```python
from build123d import *

# Parameters (mm, degrees)
F0_W         = 30
F0_H         = 10
F1_DEPTH     = 10
F2_R         = 1.75
F3_DEPTH     = 8
F4_R         = 1.75
F5_DEPTH     = 8
F6_R         = 0.5
F7_R         = 0.5
F8_T1_DEPTH  = 29
F8_T3_DEPTH  = 9
F8_T5_DEPTH  = 9
F8_S9_W      = 0.5
F8_S9_H      = 0.5
F8_T10_DEPTH = 0.5
F8_S15_W     = 0.5
F8_S15_H     = 0.5
F8_T16_DEPTH = 0.5
F8_S21_W     = 0.5
F8_S21_H     = 0.5
F8_T22_DEPTH = 0.5
F8_S27_W     = 0.5
F8_S27_H     = 0.5
F8_T28_DEPTH = 0.5
F8_T32_ANGLE = 90


# Not quite as in the source:
# - a fillet or chamfer that OpenCascade refuses, or shapes differently, is made with other operations: its cross-section is extruded or revolved along the edge and cut away or added


with BuildPart() as f1:
    # F0 (on Front) → F1 (new body)
    with BuildSketch(Plane.XZ):
        Rectangle(F0_W, F0_H)
    extrude(amount=-F1_DEPTH)

    # F2 (on face) → F3 (join)
    with BuildSketch(Plane.XY.offset(5)):
        with Locations((0, 5)):
            Circle(F2_R)
    extrude(amount=F3_DEPTH)

    # F4 (on face) → F5 (join)
    with BuildSketch(Plane(origin=(0, 0, -5), x_dir=(1, 0, 0), z_dir=(0, 0, -1))):
        with Locations((12, -5)):
            Circle(F4_R)
    extrude(amount=F5_DEPTH)

    # F6
    f6_edges = [f1.edges().sort_by_distance(p)[0] for p in [
        (0, 0, 5),
    ]]
    fillet(f6_edges, radius=F6_R)

    # F7
    f7_edges = [f1.edges().sort_by_distance(p)[0] for p in [
        (15, 5.25, 5),
        (-15, 5.25, 5),
        (0, 10, 5),
        (15, 5, -5),
        (15, 10, 0),
    ]]
    fillet(f7_edges, radius=F7_R)

    # F8: fillet of radius 0.5 on 3 edges, made by hand

    # F8_s2 → F8_t1 (cut)
    with BuildSketch(Plane.YZ.offset(-14.5)):
        with BuildLine():
            ThreePointArc((10, -4.5), (9.8535533906, -4.8535533906), (9.5, -5))
            Line((9.5, -5), (10, -5))
            Line((10, -5), (10, -4.5))
        make_face()
        with BuildLine():
            ThreePointArc((0, -4.5), (0.1464466094, -4.8535533906), (0.5, -5))
            Line((0.5, -5), (0, -5))
            Line((0, -5), (0, -4.5))
        make_face()
    extrude(amount=F8_T1_DEPTH, mode=Mode.SUBTRACT)

    # F8_s4 → F8_t3 (cut)
    with BuildSketch(Plane.XY.offset(-4.5)):
        with BuildLine():
            ThreePointArc((-15, 9.5), (-14.8535533906, 9.8535533906), (-14.5, 10))
            Line((-14.5, 10), (-15, 10))
            Line((-15, 10), (-15, 9.5))
        make_face()
    extrude(amount=F8_T3_DEPTH, mode=Mode.SUBTRACT)

    # F8_s6 → F8_t5 (cut)
    with BuildSketch(Plane.XZ.offset(-9.5)):
        with BuildLine():
            ThreePointArc((-15, -4.5), (-14.8535533906, -4.8535533906), (-14.5, -5))
            Line((-14.5, -5), (-15, -5))
            Line((-15, -5), (-15, -4.5))
        make_face()
    extrude(amount=F8_T5_DEPTH, mode=Mode.SUBTRACT)


with BuildPart() as f8_tool8:
    # F8_s9 → F8_t10 (new body)
    with BuildSketch(Plane.YZ.offset(-14.5)):
        with Locations((9.75, 4.75)):
            Rectangle(F8_S9_W, F8_S9_H)
    extrude(amount=-F8_T10_DEPTH)

    # F8_s11 → F8_t12 (revolve, cut)
    with BuildSketch(Plane(origin=(-14.5, 9.5, 4.5), x_dir=(0, -0.7071067812, -0.7071067812), z_dir=(0, 0.7071067812, -0.7071067812))):
        with BuildLine():
            ThreePointArc((0, -0.5), (0.5, 0), (0, 0.5))
            Line((0, 0.5), (0, -0.5))
        make_face()
    revolve(axis=Axis((-14.5, 9.5, 4.5), (-1, 0, 0)), mode=Mode.SUBTRACT)


with BuildPart() as f1_1:
    add(f1.part)

    # F8_t7: cut F8_tool8
    add(f8_tool8.part, mode=Mode.SUBTRACT)


with BuildPart() as f8_tool14:
    # F8_s15 → F8_t16 (new body)
    with BuildSketch(Plane.XZ.offset(-0.5)):
        with Locations((14.75, -4.75)):
            Rectangle(F8_S15_W, F8_S15_H)
    extrude(amount=F8_T16_DEPTH)

    # F8_s17 → F8_t18 (revolve, cut)
    with BuildSketch(Plane(origin=(14.5, 0.5, -4.5), x_dir=(-0.7071067812, 0, 0.7071067812), z_dir=(0.7071067812, 0, 0.7071067812))):
        with BuildLine():
            ThreePointArc((0, -0.5), (0.5, 0), (0, 0.5))
            Line((0, 0.5), (0, -0.5))
        make_face()
    revolve(axis=Axis((14.5, 0.5, -4.5), (0, -1, 0)), mode=Mode.SUBTRACT)


with BuildPart() as f1_2:
    add(f1_1.part)

    # F8_t13: cut F8_tool14
    add(f8_tool14.part, mode=Mode.SUBTRACT)


with BuildPart() as f8_tool20:
    # F8_s21 → F8_t22 (new body)
    with BuildSketch(Plane.XZ.offset(-9.5)):
        with Locations((14.75, -4.75)):
            Rectangle(F8_S21_W, F8_S21_H)
    extrude(amount=-F8_T22_DEPTH)

    # F8_s23 → F8_t24 (revolve, cut)
    with BuildSketch(Plane(origin=(14.5, 9.5, -4.5), x_dir=(-0.7071067812, 0, 0.7071067812), z_dir=(-0.7071067812, 0, -0.7071067812))):
        with BuildLine():
            ThreePointArc((0, -0.5), (0.5, 0), (0, 0.5))
            Line((0, 0.5), (0, -0.5))
        make_face()
    revolve(axis=Axis((14.5, 9.5, -4.5), (0, 1, 0)), mode=Mode.SUBTRACT)


with BuildPart() as f1_3:
    add(f1_2.part)

    # F8_t19: cut F8_tool20
    add(f8_tool20.part, mode=Mode.SUBTRACT)


with BuildPart() as f8_tool26:
    # F8_s27 → F8_t28 (new body)
    with BuildSketch(Plane.XY.offset(-4.5)):
        with Locations((-14.75, 9.75)):
            Rectangle(F8_S27_W, F8_S27_H)
    extrude(amount=-F8_T28_DEPTH)

    # F8_s29 → F8_t30 (revolve, cut)
    with BuildSketch(Plane(origin=(-14.5, 9.5, -4.5), x_dir=(0.7071067812, -0.7071067812, 0), z_dir=(0.7071067812, 0.7071067812, 0))):
        with BuildLine():
            ThreePointArc((0, -0.5), (0.5, 0), (0, 0.5))
            Line((0, 0.5), (0, -0.5))
        make_face()
    revolve(axis=Axis((-14.5, 9.5, -4.5), (0, 0, -1)), mode=Mode.SUBTRACT)


with BuildPart() as f1_4:
    add(f1_3.part)

    # F8_t25: cut F8_tool26
    add(f8_tool26.part, mode=Mode.SUBTRACT)

    # F8_s31 → F8_t32 (revolve, cut)
    with BuildSketch(Plane.YZ.offset(-14.5)):
        with BuildLine():
            ThreePointArc((0, -4.5), (0.1464466094, -4.8535533906), (0.5, -5))
            Line((0.5, -5), (0, -5))
            Line((0, -5), (0, -4.5))
        make_face()
    revolve(axis=Axis((-14.5, 0.5, -5), (0, 0, -1)), revolution_arc=F8_T32_ANGLE, mode=Mode.SUBTRACT)


solid = f1_4.part
```
Source: CAD feature listing. Evaluate the final solid. Frame: model axes, mm. A direction names the side the tool comes from. Round coordinates to 2 decimals unless told otherwise and drop trailing zeros. Loops run counter-clockwise (first coordinate to the right, second up) from the corner with the lowest first, then second, coordinate; pieces in that order, holes last. Notation, with made-up numbers: (-5.5, 51.5) - (31.5, 51.5) arc R19 cw to (31.5, 69.5) - close; hole circle Ø11 at (-33, 72.25). An arc over 180 degrees is marked (long way). Use CSV: the item, a comma, the result in double quotes.
Q1. Section query A-A, the plane y = 9. Output: boundary loops of the cut face in (x, z), then the cut area to 3 significant figures.
Reported:
outline,"(-15, -4.5) arc R0.5 ccw to (-14.5, -5) - (14.5, -5) arc R0.5 ccw to (15, -4.5) - (15, 4.5) arc R0.5 ccw to (14.5, 5) - (-14.5, 5) arc R0.5 ccw to (-15, 4.5) - close"
area,"300 mm^2"
Q2. Section query D-D, the plane y = 5. Output: boundary loops of the cut face in (x, z).
Reported:
outline,"(-15, -4.5) arc R0.5 ccw to (-14.5, -5) - (10.25, -5) - (10.25, -13) - (13.75, -13) - (13.75, -5) - (14.5, -5) arc R0.5 ccw to (15, -4.5) - (15, 4.5) arc R0.5 ccw to (14.5, 5) - (1.75, 5) - (1.75, 13) - (-1.75, 13) - (-1.75, 5) - (-14.5, 5) arc R0.5 ccw to (-15, 4.5) - close"
Q3. Section query C-C, the plane z = 11.25. Output: boundary loops of the cut face in (x, y), then the cut area to 3 significant figures.
Reported:
outline,"circle Ø3.5 at (0, 5)"
area,"9.62 mm^2"
Q4. Pin query (flat end, axial travel): pin 1 Ø3 at (x, y) = (4, 6.5) entering from +Z; pin 2 Ø6 at (x, z) = (4.5, -6.5) entering from -Y; pin 3 Ø5 at (x, y) = (-3.5, 2) entering from -Z; pin 4 Ø4 at (y, z) = (6, -9.5) entering from -X. Return the tip coordinate at first contact, or that it passes through.
Reported:
pin 1,"z = 5"
pin 2,"y = 0"
pin 3,"z = -5"
pin 4,"x = 10.25"
Q5. Section query B-B, the plane x = -5. Output: boundary loops of the cut face in (y, z), then the cut area to 3 significant figures.
Reported:
outline,"(0, -4.5) arc R0.5 ccw to (0.5, -5) - (9.5, -5) arc R0.5 ccw to (10, -4.5) - (10, 4.5) arc R0.5 ccw to (9.5, 5) - (0.5, 5) arc R0.5 ccw to (0, 4.5) - close"
area,"99.8 mm^2"
Q6. Ray query, line 1 along Z through (x, y) = (-8, 4.75); line 2 along X through (y, z) = (3.5, 8); line 3 along Y through (x, z) = (13, 4.75). Return the intervals inside material, ascending.
Reported:
line 1,"-5 to 5"
line 2,"-0.9 to 0.9"
line 3,"0.07 to 9.93"
Q7. Reachability of faces 1 (the cylindrical face through (13.617, 5.67, -8.944)), 2 (the cylindrical face through (-0.38, 3.29, 8.94)), 3 (the flat face through (12, 5, -13)) from +Z, -Z, +X, -X, +Y, -Y: full face, straight path, thin tool, end or side. Return the list, or none.
Reported:
face 1,"-Z"
face 2,"+Z"
face 3,"-Z, +X, -X, +Y, -Y"
